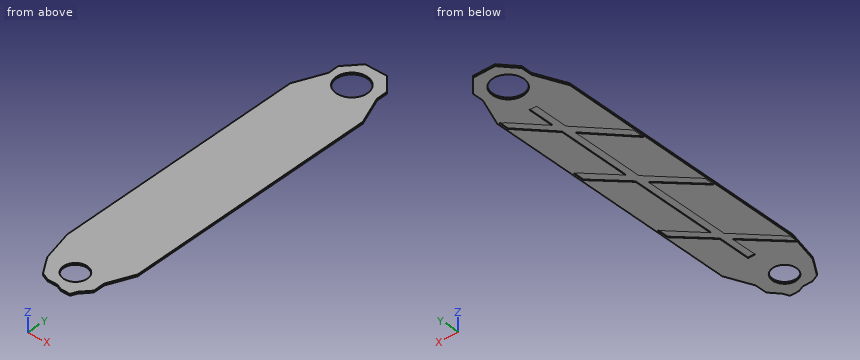
```python
from build123d import *

# Parameters (mm, degrees)
F2_DEPTH = 0.762
F3_D     = 13.335
F4_D     = 10.16
F6_DEPTH = 0.2286


with BuildPart() as f2:
    # F1 (on Top) → F2 (new body)
    with BuildSketch(Plane.XY):
        Polygon((5.1344926469, 79.8476114869), (0, 79.8476114869), (-4.2268559337, 79.8476114869), (-7.4234125204, 76.1947035789), (-9.9349934608, 73.4550207853), (-9.9349934608, 68.6605796218), (-15.4148070142, 56.3320219517), (-15.4148070142, -51.4287278056), (-12.2182490304, -64.6705105901), (-9.9349934608, -68.323418498), (-7.4234125204, -72.2046345472), (-4.2268559337, -73.6254442297), (0, -73.6254442297), (2.4043139854, -74.6941168771), (6.2761204317, -74.6941168771), (7.382648817, -72.2046345472), (10.842631571, -68.323418498), (10.842631571, -63.3006691933), (15.6444913902, -52.4973808827), (15.6444913902, -7.1372324601), (15.6444913902, 14.5519021899), (15.6444913902, 38.0674898624), (15.6444913902, 52.4508096278), (15.6444913902, 56.3320219517), (10.842631571, 68.6605796218), (10.842631571, 73.4550207853), align=None)
    extrude(amount=F2_DEPTH)

    # F3 (through all)
    with Locations(Plane(origin=(0, 0, 0), x_dir=(1, 0, 0), z_dir=(0, 0, -1))):
        with Locations((0, -68.7236785889)):
            Hole(F3_D / 2)

    # F4 (through all)
    with Locations(Plane(origin=(0, 0, 0), x_dir=(1, 0, 0), z_dir=(0, 0, -1))):
        with Locations((0, 64.9243146181)):
            Hole(F4_D / 2)

    # F5 (on Top) → F6 (cut)
    with BuildSketch(Plane.XY):
        Polygon((14.8983420804, 55.9992268682), (13.3339157328, 55.0209134817), (3.0205850489, 43.9974281211), (3.0205850489, 39.1634636204), (14.8983420804, 51.9865565002), align=None)
        Polygon((3.0205850489, 39.1634636204), (3.0205850489, 43.9974281211), (0, 40.7688518165), (0, 35.9024739797), align=None)
        Polygon((0, 40.7688518165), (3.0205850489, 43.9974281211), (3.0205850489, 55.0209134817), (0, 55.0209134817), align=None)
        Polygon((0, 35.9024739797), (0, 40.7688518165), (-14.7966286168, 24.9533578753), (-14.7966286168, 19.9282001704), align=None)
        Polygon((3.0205850489, 8.5766670856), (3.0205850489, 39.1634636204), (0, 35.9024739797), (0, 5.5005631668), align=None)
        Polygon((3.0205850489, 3.6877155311), (3.0205850489, 8.5766670856), (0, 5.5005631668), (0, 0.6926685426), align=None)
        Polygon((13.3339157328, 19.0795585513), (3.0205850489, 8.5766670856), (3.0205850489, 3.6877155311), (14.8983420804, 15.4650500044), (14.8983420804, 20.2802531421), align=None)
        Polygon((0, 0.6926685426), (0, 5.5005631668), (-14.7966286168, -9.5680300146), (-14.7966286168, -13.9788594097), align=None)
        Polygon((3.0205850489, -32.5537367418), (3.0205850489, 3.6877155311), (0, 0.6926685426), (0, -35.6298406606), align=None)
        Polygon((3.0205850489, -37.0688434684), (3.0205850489, -32.5537367418), (0, -35.6298406606), (0, -40.0638904568), align=None)
        Polygon((14.8983420804, -20.4576645046), (3.0205850489, -32.5537367418), (3.0205850489, -37.0688434684), (14.8983420804, -25.291508995), align=None)
        Polygon((0, -40.0638904568), (0, -35.6298406606), (-14.7966286168, -50.698433842), (-14.7966286168, -54.7354184091), align=None)
        Polygon((3.0205850489, -50.698433842), (3.0205850489, -37.0688434684), (0, -40.0638904568), (0, -50.698433842), align=None)
    extrude(amount=F6_DEPTH, mode=Mode.SUBTRACT)


solid = f2.part
```
Geometry: final body of the model. Coordinates: model frame, mm. Give positions to 0.01 mm unless a question says otherwise; leave off trailing zeros. Order: outer loops, then holes, each group sorted by start corner. A loop starts at its lowest first (then second) coordinate and runs counter-clockwise, first axis right, second up. Notation, with made-up numbers: M -22,40.25 L 20,40.25 A25 ccw 20,53.25 Z; hole C -23.5,-22 d3. An arc over 180 degrees is marked long. Answer as CSV lines item,"result". Start each with the question number.
1) Cut plane C-C (y = -44). Output: boundary loops of the cut face in (x, z).
2) Line query: line 1 (Y direction, x = 0, z = 0.65); line 2 (Y direction, x = 3, z = 0.7); line 3 (Z direction, x = -10, y = 28.5). Output: solid intervals per line, ascending. Write a range as from..to.
3) Cut plane A-A (z = 0.55). Output: boundary loops of the cut face in (x, y) (1 decimal), then the cut area to 3 significant figures.
4) Cut plane B-B (y = 29.5). Output: boundary loops of the cut face in (x, z).
Findings below:
1,outline,"M -15.41,0 L -8.22,0 L -8.22,0.23 L -3.97,0.23 L -3.97,0 L 0,0 L 0,0.23 L 3.02,0.23 L 3.02,0 L 15.64,0 L 15.64,0.76 L -15.41,0.76 Z"
2,line 1,"y = -73.63..-70, -59.84..62.06, 75.39..79.85"
2,line 2,"y = -74.69..-69.02, -60.82..62.77, 74.68..79.85"
2,line 3,"z = 0.23..0.76"
3,outline,"M -15.4,-51.4 L -12.2,-64.7 L -9.9,-68.3 L -7.4,-72.2 L -4.2,-73.6 L 0,-73.6 L 2.4,-74.7 L 6.3,-74.7 L 7.4,-72.2 L 10.8,-68.3 L 10.8,-63.3 L 15.6,-52.5 L 15.6,56.3 L 10.8,68.7 L 10.8,73.5 L 5.1,79.8 L -4.2,79.8 L -7.4,76.2 L -9.9,73.5 L -9.9,68.7 L -15.4,56.3 Z; hole C 0,68.7 d13.3; hole C 0,-64.9 d10.2"
3,area,"4,170 mm²"
4,outline,"M -15.41,0 L -10.54,0 L -10.54,0.23 L -5.93,0.23 L -5.93,0 L 0,0 L 0,0.23 L 3.02,0.23 L 3.02,0 L 15.64,0 L 15.64,0.76 L -15.41,0.76 Z"
